CAD build for the part. Positions are in the model's coordinates, mm. A direction names the side the tool comes from. Give positions to 0.01 mm unless a question says otherwise; leave off trailing zeros. Loops run counter-clockwise (first coordinate to the right, second up) from the corner with the lowest first, then second, coordinate; pieces in that order, holes last.
```python
from build123d import *

# Parameters (mm, degrees)
SKETCH001_R        = 2.1
HOLE_DEPTH         = 233.001
POLARPATTERN_COUNT = 4


with BuildPart() as part:
    # Sketch → Revolution (revolve)
    with BuildSketch(Plane.XZ):
        Polygon((0, 11.5), (14, 11.5), (14, 40), (9, 40), (9, 19), (0, 19), align=None)
    revolve(axis=Axis((0, 0, 0), (1, 0, 0)))

    # Sketch001 (on Face4 of Revolution) → Hole (cut, through all)
    with BuildSketch(Plane(origin=(9, 0, 0), x_dir=(0, 0, -1), z_dir=(-1, 0, 0))):
        with Locations((30, 0)):
            Circle(SKETCH001_R)
    hole = extrude(amount=-HOLE_DEPTH, mode=Mode.SUBTRACT)

    # PolarPattern: Hole ×4 about axis
    polarpattern_axis = Axis((9, 0, 0), (-1, 0, 0))
    for i in range(1, POLARPATTERN_COUNT):
        add(hole.rotate(polarpattern_axis, i * 360 / POLARPATTERN_COUNT), mode=Mode.SUBTRACT)


solid = part.part
```
1. Saw through at A-A, the plane y = 0. List the corners of the cut face in (x, z).
Responses:
outline: (0, -19) - (9, -19) - (9, -27.9) - (14, -27.9) - (14, -11.5) - (0, -11.5) - close; (0, 11.5) - (14, 11.5) - (14, 27.9) - (9, 27.9) - (9, 19) - (0, 19) - close; (9, -40) - (14, -40) - (14, -32.1) - (9, -32.1) - close; (9, 32.1) - (14, 32.1) - (14, 40) - (9, 40) - close
2. Saw through at C-C, the plane x = 12.5. List the corners of the cut face in (y, z), and give its area (3 significant figures).
Responses:
outline: circle Ø80 at (0, 0); hole circle Ø4.2 at (-30, 0); hole circle Ø23 at (0, 0); hole circle Ø4.2 at (0, -30); hole circle Ø4.2 at (0, 30); hole circle Ø4.2 at (30, 0)
area: 4,560 mm2
3. Tool access for faces 1 (the face through (11.46, 0.09, 27.9)), 2 (the face through (9, -9, 17)): list every direction of +Z, -Z, +X, -X, +Y, -Y with a clear straight run to the whole face (end or side of a thin tool).
Responses:
face 1: +X, -X
face 2: -X
4. Saw through at D-D, the plane y = -29. List the corners of the cut face in (x, z), and give its area (3 significant figures).
Responses:
outline: (9, -27.55) - (14, -27.55) - (14, -1.85) - (9, -1.85) - close; (9, 1.85) - (14, 1.85) - (14, 27.55) - (9, 27.55) - close
area: 257 mm2
5. Pull direction Y, two halves, no side cores. Call faces 3 (the face through (11.46, -0.09, -27.9)), 4 (the face through (4.437, 16.856, 8.767)), 5 (the face through (14, 8.3, -8.3)): released by +Y, released by -Y, zero draft, split by the parting line, or undercut.
Responses:
face 3: undercut
face 4: split by the parting line
face 5: zero draft
6. Drop flat-ended pins along their axis: pin 1 (2 mm diameter, centred on x = 9.5, y = 30, fed in from -Z); pin 2 (5.5 mm diameter, centred on y = 0, z = 30, fed in from -X); pin 3 (2 mm diameter, centred on x = 12.5, z = 26, fed in from -Y) (3 decimals). Give the stop position or say it passes through.
Responses:
pin 1: stops at z = -27.55
pin 2: stops at x = 9
pin 3: stops at y = -31.225
7. Probe line 1 along X through (y, z) = (29.5, 7); line 2 along Z through (x, y) = (10.5, -5); line 3 along Z through (x, y) = (13, 9.5). List the from-to ranges inside material, lowest first.
Responses:
line 1: x = 9 to 14
line 2: z = -39.69 to -10.36, 10.36 to 39.69
line 3: z = -38.86 to -6.48, 6.48 to 38.86
